Model file for the job. Use its own axes, mm. A direction names the side the tool comes from. Round coordinates to 2 decimals unless told otherwise and drop trailing zeros. Loops run counter-clockwise (first coordinate to the right, second up) from the corner with the lowest first, then second, coordinate; pieces in that order, holes last. Notation, with made-up numbers: (35, 61.5) -> (84, 61.5) arc R28 cw to (84, 82.5) -> close; hole circle Ø8 at (73.5, 26.25). An arc over 180 degrees is marked (long way). Use a Markdown table: item, result. Add a question column.
```python
from build123d import *

# Parameters (mm, degrees)
SKETCH1_R           = 6.8961
SKETCH1_R_2         = 2.3241
BOSS_EXTRUDE1_DEPTH = 2.794
SKETCH2_R           = 2.3241
BOSS_EXTRUDE2_DEPTH = 0.254
BOSS_EXTRUDE3_DEPTH = 1.651
BOSS_EXTRUDE4_START = 2.286
SKETCH4_R           = 6.8961
BOSS_EXTRUDE4_DEPTH = 2.286
FILLET1_R           = 0.254
FILLET2_R           = 0.127
FILLET3_R           = 0.4


with BuildPart() as part:
    # Sketch1 → Boss-Extrude1 (new body)
    with BuildSketch(Plane(origin=(0, 0, 0), x_dir=(1, 0, 0), z_dir=(0, 1, 0))):
        with Locations(Location((0, 0, 0), (0, 0, 270))):
            Circle(SKETCH1_R)
        with Locations(Location((0, 0, 0), (0, 0, 270))):
            Circle(SKETCH1_R_2, mode=Mode.SUBTRACT)
    extrude(amount=BOSS_EXTRUDE1_DEPTH)

    # Sketch2 → Boss-Extrude2 (add)
    with BuildSketch(Plane.XZ):
        with Locations(Location((0, 0, 0), (0, 0, 270))):
            Circle(SKETCH2_R)
    extrude(amount=-BOSS_EXTRUDE2_DEPTH)

    # Sketch3 → Boss-Extrude3 (add)
    with BuildSketch(Plane(origin=(0, 0.254, 0), x_dir=(1, 0, 0), z_dir=(0, 1, 0))):
        with BuildLine():
            Line((-0.495805164, 1.156686678), (0.614449488, 1.120298857))
            ThreePointArc((0.614449488, 1.120298857), (0.708812351, 1.091670316), (0.776218716, 1.01969584))
            Line((0.776218716, 1.01969584), (1.299833265, 0.039993196))
            ThreePointArc((1.299833265, 0.039993196), (1.322221652, -0.056041711), (1.293593111, -0.150404573))
            Line((1.293593111, -0.150404573), (0.706953007, -1.093719397))
            ThreePointArc((0.706953007, -1.093719397), (0.634978532, -1.161125762), (0.538943625, -1.183514149))
            Line((0.538943625, -1.183514149), (-0.571311028, -1.147126328))
            ThreePointArc((-0.571311028, -1.147126328), (-0.66567389, -1.118497787), (-0.733080255, -1.046523312))
            Line((-0.733080255, -1.046523312), (-1.256694804, -0.066820667))
            ThreePointArc((-1.256694804, -0.066820667), (-1.279083191, 0.02921424), (-1.25045465, 0.123577102))
            Line((-1.25045465, 0.123577102), (-0.663814546, 1.066891925))
            ThreePointArc((-0.663814546, 1.066891925), (-0.591840071, 1.134298291), (-0.495805164, 1.156686678))
        make_face()
    extrude(amount=BOSS_EXTRUDE3_DEPTH)

    # Sketch4 → Boss-Extrude4 (add)
    with BuildSketch(Plane.XZ.offset(BOSS_EXTRUDE4_START)):
        with Locations(Location((0, 0, 0), (0, 0, 270))):
            Circle(SKETCH4_R)
    extrude(amount=-BOSS_EXTRUDE4_DEPTH)

    # Fillet1
    fillet1_edges = [part.edges().sort_by_distance(p)[0] for p in [
        (0, 0.254, -2.3241),
        (0.708812351, 0.254, -1.091670316),
        (0.059322162, 0.254, -1.138492768),
        (-0.591840071, 0.254, -1.134298291),
        (-0.957134598, 0.254, -0.595234514),
        (-1.279083191, 0.254, -0.02921424),
        (-0.99488753, 0.254, 0.556671989),
        (-0.66567389, 0.254, 1.118497787),
        (-0.016183701, 0.254, 1.165320239),
        (0.634978532, 0.254, 1.161125762),
        (1.000273059, 0.254, 0.622061985),
        (1.322221652, 0.254, 0.056041711),
        (1.038025991, 0.254, -0.529844518),
    ]]
    fillet(fillet1_edges, radius=FILLET1_R)

    # Fillet2
    fillet2_edges = [part.edges().sort_by_distance(p)[0] for p in [
        (0.708812351, 1.905, -1.091670316),
        (0.059322162, 1.905, -1.138492768),
        (-0.591840071, 1.905, -1.134298291),
        (-0.957134598, 1.905, -0.595234514),
        (-1.279083191, 1.905, -0.02921424),
        (-0.99488753, 1.905, 0.556671989),
        (-0.66567389, 1.905, 1.118497787),
        (-0.016183701, 1.905, 1.165320239),
        (0.634978532, 1.905, 1.161125762),
        (1.000273059, 1.905, 0.622061985),
        (1.322221652, 1.905, 0.056041711),
        (1.038025991, 1.905, -0.529844518),
    ]]
    fillet(fillet2_edges, radius=FILLET2_R)

    # Fillet3
    fillet3_edges = [part.edges().sort_by_distance(p)[0] for p in [
        (0, 2.794, -6.8961),
    ]]
    fillet(fillet3_edges, radius=FILLET3_R)


solid = part.part
```
1) Wall check: probe 1 along Z at (x, y) = (0, 1.55); probe 2 along Z at (x, y) = (0, 2.15). Give the ranges that are in metal, low to high. Write a range as from..to.
2) Cut at A-A on y = -1.05. Write the cut outline in (x, z).
3) Pin check, flat tips, straight feed: pin 1 Ø0.6 at (x, z) = (0, 0.5) entering from +Y (3 decimals); pin 2 Ø3 at (x, y) = (2, 1.5) entering from +Z; pin 3 Ø1 at (y, z) = (-1.5, -1) entering from -X; pin 4 Ø4.5 at (x, z) = (0.5, -0.5) entering from +Y. Stop position of each tip, or through.
4) Tool access for faces 3 (the face through (1.034, 1.134, -0.537)), 4 (the face through (0, -2.286, 0)): list every direction of +Z, -Z, +X, -X, +Y, -Y with a clear straight run to the whole face (end or side of a thin tool).
5) Pull direction Z, two halves, no side cores. Call faces 1 (the face through (-0.96, 1.13, -0.59)), 2 (the face through (0, 2.794, 3)): +Z half, -Z half, draft (parallel to the pull), parting line (faces both ways), or undercut.
Established:
| question | item | result |
|---|---|---|
| 1 | probe 1 | z = -6.9..-2.32, -1.14..1.17, 2.32..6.9 |
| 1 | probe 2 | z = -6.9..-2.32, 2.32..6.9 |
| 2 | outline | circle Ø13.79 at (0, 0) |
| 3 | pin 1 | stops at y = 1.905 |
| 3 | pin 2 | stops at z = 6.88 |
| 3 | pin 3 | stops at x = -6.88 |
| 3 | pin 4 | stops at y = 2.79 |
| 4 | face 3 | +Y |
| 4 | face 4 | +Z, -Z, +X, -X, -Y |
| 5 | face 1 | undercut |
| 5 | face 2 | draft |
